```python
from build123d import *

# Parameters (mm, degrees)
SKETCH1_W           = 85
SKETCH1_H           = 56.25
BOSS_EXTRUDE1_DEPTH = 1.5
SKETCH2_W           = 6.5
SKETCH2_H           = 6.5
BOSS_EXTRUDE2_DEPTH = 3
SKETCH3_R           = 1.175
BOSS_EXTRUDE3_DEPTH = 5
SKETCH4_W           = 56.25
SKETCH4_H           = 1.5
BOSS_EXTRUDE4_DEPTH = 5
BOSS_EXTRUDE5_DEPTH = 11
SKETCH6_W           = 90
SKETCH6_H           = 3
BOSS_EXTRUDE6_DEPTH = 12.5
SKETCH7_W           = 6
SKETCH7_H           = 3
SKETCH7_W_2         = 9
SKETCH7_W_3         = 16
SKETCH7_W_4         = 7.5
SKETCH7_W_5         = 3
SKETCH7_H_2         = 16
CUT_EXTRUDE1_DEPTH  = 6.5
CUT_EXTRUDE2_DEPTH  = 6.5
SKETCH9_W           = 6.5
SKETCH9_H           = 43.25
BOSS_EXTRUDE7_DEPTH = 1
SKETCH10_W          = 9.5
SKETCH10_H          = 1
CUT_EXTRUDE3_DEPTH  = 0.5
SKETCH11_W          = 11
SKETCH11_H          = 1
CUT_EXTRUDE4_DEPTH  = 4
SKETCH12_W          = 8
SKETCH12_H          = 1
CUT_EXTRUDE5_DEPTH  = 1
SKETCH13_W          = 0.75
SKETCH13_H          = 56.25
CUT_EXTRUDE6_DEPTH  = 8


with BuildPart() as part:
    # Sketch1 → Boss-Extrude1 (new body)
    with BuildSketch(Plane(origin=(0, 0, 0), x_dir=(1, 0, 0), z_dir=(0, 1, 0))):
        with Locations((42.5, 28.125)):
            Rectangle(SKETCH1_W, SKETCH1_H)
    extrude(amount=BOSS_EXTRUDE1_DEPTH)

    # Sketch2 → Boss-Extrude2 (add)
    with BuildSketch(Plane(origin=(0, 1.5, 0), x_dir=(1, 0, 0), z_dir=(0, 1, 0))):
        with Locations((3.25, 3.25)):
            Rectangle(SKETCH2_W, SKETCH2_H)
        with Locations((61.5, 3.25)):
            Rectangle(SKETCH2_W, SKETCH2_H)
        with Locations((61.5, 53)):
            Rectangle(SKETCH2_W, SKETCH2_H)
        with Locations((3.25, 53)):
            Rectangle(SKETCH2_W, SKETCH2_H)
    extrude(amount=BOSS_EXTRUDE2_DEPTH)

    # Sketch3 → Boss-Extrude3 (add)
    with BuildSketch(Plane(origin=(0, 4.5, 0), x_dir=(1, 0, 0), z_dir=(0, 1, 0))):
        with Locations(Location((3.5, 3.5, 0), (0, 0, 90))):
            Circle(SKETCH3_R)
        with Locations(Location((61.5, 3.5, 0), (0, 0, 90))):
            Circle(SKETCH3_R)
        with Locations(Location((61.5, 52.75, 0), (0, 0, 90))):
            Circle(SKETCH3_R)
        with Locations(Location((3.5, 52.75, 0), (0, 0, 90))):
            Circle(SKETCH3_R)
    extrude(amount=BOSS_EXTRUDE3_DEPTH)

    # Sketch4 → Boss-Extrude4 (add)
    with BuildSketch(Plane.ZY):
        with Locations((-28.125, 0.75)):
            Rectangle(SKETCH4_W, SKETCH4_H)
    extrude(amount=BOSS_EXTRUDE4_DEPTH)

    # Sketch5 → Boss-Extrude5 (add)
    with BuildSketch(Plane(origin=(0, 1.5, 0), x_dir=(1, 0, 0), z_dir=(0, 1, 0))):
        Polygon((-5, 0), (-2.5, 0), (0, 0), (0, 6.5), (-2, 6.5), (-2, 49.75), (0, 49.75), (0, 56.25), (-2.5, 56.25), (-5, 56.25), align=None)
    extrude(amount=BOSS_EXTRUDE5_DEPTH)

    # Sketch6 → Boss-Extrude6 (add)
    with BuildSketch(Plane(origin=(0, 0, 0), x_dir=(1, 0, 0), z_dir=(0, 1, 0))):
        with Locations((40, -1.5)):
            Rectangle(SKETCH6_W, SKETCH6_H)
        Polygon((85, 56.25), (85, 0), (85, -3), (88, -3), (88, 56.25), align=None)
        Polygon((-5, 56.25), (85, 56.25), (88, 56.25), (88, 59.25), (-5, 59.25), align=None)
    extrude(amount=BOSS_EXTRUDE6_DEPTH)

    # Sketch7 → Cut-Extrude1 (cut)
    with BuildSketch(Plane(origin=(0, 12.5, 0), x_dir=(1, 0, 0), z_dir=(0, 1, 0))):
        with Locations((12, 57.75)):
            Rectangle(SKETCH7_W, SKETCH7_H)
        Polygon((86.5, 40), (86.5, 38.5), (88, 38.5), (88, 55), (86.5, 55), (86.5, 53.5), (85, 53.5), (85, 40), align=None)
        with Locations((10.5, -1.5)):
            Rectangle(SKETCH7_W_2, SKETCH7_H)
        with Locations((32, -1.5)):
            Rectangle(SKETCH7_W_3, SKETCH7_H)
        with Locations((53.75, -1.5)):
            Rectangle(SKETCH7_W_4, SKETCH7_H)
        with Locations((86.5, 10.25)):
            Rectangle(SKETCH7_W_5, SKETCH7_H_2)
        Polygon((86.5, 35.75), (86.5, 37.25), (88, 37.25), (88, 20.75), (86.5, 20.75), (86.5, 22.25), (85, 22.25), (85, 35.75), align=None)
    extrude(amount=-CUT_EXTRUDE1_DEPTH, mode=Mode.SUBTRACT)

    # Sketch8 → Cut-Extrude2 (cut)
    with BuildSketch(Plane.ZY.offset(5)):
        Polygon((-35.625, 0), (-20.625, 0), (-19.125, 1.5), (-20.625, 1.5), (-20.625, 5.5), (-35.625, 5.5), (-35.625, 1.5), (-37.125, 1.5), align=None)
    extrude(amount=-CUT_EXTRUDE2_DEPTH, mode=Mode.SUBTRACT)

    # Sketch9 → Boss-Extrude7 (add)
    with BuildSketch(Plane(origin=(0, 1.5, 0), x_dir=(1, 0, 0), z_dir=(0, 1, 0))):
        with Locations((61.5, 28.125)):
            Rectangle(SKETCH9_W, SKETCH9_H)
    extrude(amount=BOSS_EXTRUDE7_DEPTH)

    # Sketch10 → Cut-Extrude3 (cut)
    with BuildSketch(Plane(origin=(0, 12.5, 0), x_dir=(1, 0, 0), z_dir=(0, 1, 0))):
        with Locations((53.75, -1.5)):
            Rectangle(SKETCH10_W, SKETCH10_H)
    extrude(amount=-CUT_EXTRUDE3_DEPTH, mode=Mode.SUBTRACT)

    # Sketch11 → Cut-Extrude4 (cut)
    with BuildSketch(Plane(origin=(0, 12.5, 0), x_dir=(1, 0, 0), z_dir=(0, 1, 0))):
        with Locations((10.5, -1.5)):
            Rectangle(SKETCH11_W, SKETCH11_H)
    extrude(amount=-CUT_EXTRUDE4_DEPTH, mode=Mode.SUBTRACT)

    # Sketch12 → Cut-Extrude5 (cut)
    with BuildSketch(Plane(origin=(0, 12.5, 0), x_dir=(1, 0, 0), z_dir=(0, 1, 0))):
        with Locations((12, 57.75)):
            Rectangle(SKETCH12_W, SKETCH12_H)
    extrude(amount=-CUT_EXTRUDE5_DEPTH, mode=Mode.SUBTRACT)

    # Sketch13 → Cut-Extrude6 (cut)
    with BuildSketch(Plane(origin=(0, 12.5, 0), x_dir=(1, 0, 0), z_dir=(0, 1, 0))):
        with Locations((-0.375, 28.125)):
            Rectangle(SKETCH13_W, SKETCH13_H)
    extrude(amount=-CUT_EXTRUDE6_DEPTH, mode=Mode.SUBTRACT)


solid = part.part
```
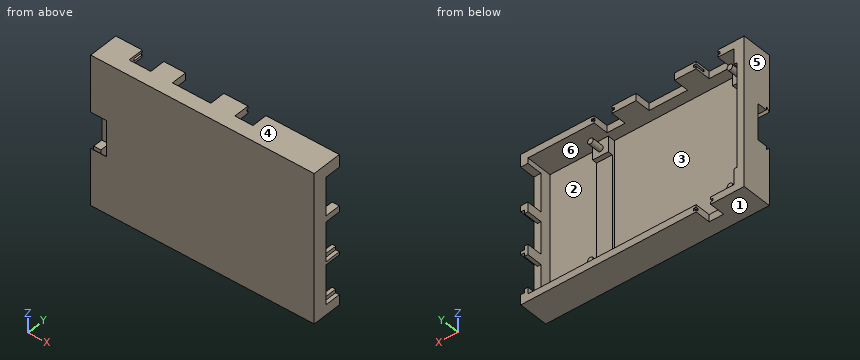
Source: CAD feature listing. Evaluate the final solid. Frame: model axes, mm. Face numbers are marked on the shaded views. A direction names the side the tool comes from. Coordinates: 2 decimals unless noted, no trailing zeros. Write each loop counter-clockwise with the first axis right and the second up, starting at its lowest first coordinate (ties: lowest second). Pieces come first, ordered by that corner, then holes. Notation, with made-up numbers: (56.25, 58.25) -> (88.25, 58.25) arc R32 ccw to (88.25, 87.25) -> close; hole circle Ø5 at (5, 86). An arc over 180 degrees is marked (long way). Return JSON: item names as keys, results as strings. Group by question number.
1) Section query A-A, the plane x = 35. Return loops of the section in (y, z), plus the area to 3 significant figures.
2) Section query B-B, the plane z = -46. Return loops of the section in (x, y).
3) Mould query, pull axis X, two halves, no side actions, for the marked faces 3, 4, 5 and 6. Classes: +X half, -X half, draft (parallel to the pull), parting line (faces both ways), or undercut.
4) Contact query for flat-ended pins moving along their axis: P1, Ø10, axis at x = 68, z = -26.5, coming from the +Y side; P2, Ø5, axis at x = 21, z = -17.5, coming from the +Y side; P3, Ø0.9, axis at x = 86, z = -30.5, coming from the +Y side. Output: stop coordinate, or through.
5) Ray query, line 1 along Z through (x, y) = (37.5, 3.75); line 2 along Z through (x, y) = (62.5, 3); line 3 along Y through (x, z) = (82, -45). Return the intervals inside material, ascending.
6) Set-up query: the marked faces 1 and 2. Return all of +Z, -Z, +X, -X, +Y, -Y with unobstructed straight access to the full face (end or side cutting, diameter ignored); none if empty.
7) Section query D-D, the plane x = 3.5. Return loops of the section in (y, z) (3 decimals).
8) Section query C-C, the plane y = 10.5. State how many separate pieces and enclosed holes the cut face has, plus the area to 3 significant figures.
From the geometry:
{
 "1": {"outline": "(0, -59.25) -> (12.5, -59.25) -> (12.5, -56.25) -> (1.5, -56.25) -> (1.5, 0) -> (6, 0) -> (6, 3) -> (0, 3) -> close", "area": "140 mm²"},
 "2": {"outline": "(-5, 0) -> (88, 0) -> (88, 6) -> (85, 6) -> (85, 1.5) -> (64.75, 1.5) -> (64.75, 2.5) -> (58.25, 2.5) -> (58.25, 1.5) -> (-2, 1.5) -> (-2, 12.5) -> (-5, 12.5) -> close"},
 "3": {"face 3": "undercut", "face 4": "draft", "face 5": "-X half", "face 6": "undercut"},
 "4": {"P1": "y = 2.5", "P2": "y = 1.5", "P3": "y = 6"},
 "5": {"line 1": "-59.25 to -56.25, 0 to 3", "line 2": "-59.25 to -49.75, -6.5 to 3", "line 3": "0 to 1.5"},
 "6": {"face 1": "-Z, +X, -X, +Y, -Y", "face 2": "+Y"},
 "7": {"outline": "(0, -59.25) -> (12.5, -59.25) -> (12.5, -56.25) -> (4.5, -56.25) -> (4.5, -53.925) -> (9.5, -53.925) -> (9.5, -51.575) -> (4.5, -51.575) -> (4.5, -49.75) -> (1.5, -49.75) -> (1.5, -6.5) -> (4.5, -6.5) -> (4.5, -4.675) -> (9.5, -4.675) -> (9.5, -2.325) -> (4.5, -2.325) -> (4.5, 0) -> (12.5, 0) -> (12.5, 3) -> (0, 3) -> close"},
 "8": {"separate pieces": "7", "enclosed holes": "0", "area": "656 mm²"}
}
